Check sheet for the modelled part. Datum: model origin and axes. Units: mm. A direction names the side the tool comes from. Coordinates: 2 decimals unless noted, no trailing zeros. Loops run counter-clockwise (first coordinate to the right, second up) from the corner with the lowest first, then second, coordinate; pieces in that order, holes last. Notation, with made-up numbers: M -5,59.5 L -1,59.5 A16 ccw -1,68.5 Z; hole C 24,-22.75 d6. An arc over 180 degrees is marked long. Return JSON: item names as keys, results as strings.
from build123d import *

# Parameters (mm, degrees)
SKETCH_R      = 1.5
PAD_DEPTH     = 2.5
SKETCH001_R   = 4.25
PAD001_DEPTH  = 2.8
SKETCH002_R   = 15
PAD002_DEPTH  = 14.9
SKETCH003_R   = 2.5
PAD003_DEPTH  = 15
CHAMFER_SIZE2 = 6
CHAMFER_SIZE  = 4
SKETCH004_R   = 5
POCKET_DEPTH  = 1
SKETCH005_R   = 4
PAD004_DEPTH  = 1
SKETCH006_R   = 2
PAD005_DEPTH  = 0.95


with BuildPart() as part:
    # Sketch → Pad (new body)
    with BuildSketch(Plane.XY):
        with BuildLine():
            ThreePointArc((2.946794, 7.4375), (0, 11), (-2.946794, 7.4375))
            ThreePointArc((-3.519561, 5.765095), (-2.886811, 6.482674), (-2.946794, 7.4375))
            ThreePointArc((-3.519561, 5.765095), (-4.776172, 4.776172), (-5.765095, 3.519561))
            ThreePointArc((-7.4375, 2.946794), (-6.482674, 2.886811), (-5.765095, 3.519561))
            ThreePointArc((-7.4375, 2.946794), (-11, 0), (-7.4375, -2.946794))
            ThreePointArc((-5.765095, -3.519561), (-6.482674, -2.886811), (-7.4375, -2.946794))
            ThreePointArc((-5.765095, -3.519561), (-4.776172, -4.776172), (-3.519561, -5.765095))
            ThreePointArc((-2.946794, -7.4375), (-2.886811, -6.482674), (-3.519561, -5.765095))
            ThreePointArc((-2.946794, -7.4375), (0, -11), (2.946794, -7.4375))
            ThreePointArc((3.519561, -5.765095), (2.886811, -6.482674), (2.946794, -7.4375))
            ThreePointArc((3.519561, -5.765095), (4.776172, -4.776172), (5.765095, -3.519561))
            ThreePointArc((7.4375, -2.946794), (6.482674, -2.886811), (5.765095, -3.519561))
            ThreePointArc((7.4375, -2.946794), (11, 0), (7.4375, 2.946794))
            ThreePointArc((5.765095, 3.519561), (6.482674, 2.886811), (7.4375, 2.946794))
            ThreePointArc((5.765095, 3.519561), (4.776172, 4.776172), (3.519561, 5.765095))
            ThreePointArc((2.946794, 7.4375), (2.886811, 6.482674), (3.519561, 5.765095))
        make_face()
        with Locations((0, 8)):
            Circle(SKETCH_R, mode=Mode.SUBTRACT)
        with Locations((8, 0)):
            Circle(SKETCH_R, mode=Mode.SUBTRACT)
        with Locations((0, -8)):
            Circle(SKETCH_R, mode=Mode.SUBTRACT)
        with Locations((-8, 0)):
            Circle(SKETCH_R, mode=Mode.SUBTRACT)
    extrude(amount=PAD_DEPTH)

    # Sketch001 (on Face22 of Pad) → Pad001 (join)
    with BuildSketch(Plane.XY.offset(2.5)):
        Circle(SKETCH001_R)
    extrude(amount=PAD001_DEPTH)

    # Sketch002 (on Face24 of Pad001) → Pad002 (join)
    with BuildSketch(Plane.XY.offset(5.3)):
        Circle(SKETCH002_R)
    extrude(amount=PAD002_DEPTH)

    # Sketch003 (on Face3 of Pad002) → Pad003 (join)
    with BuildSketch(Plane.XY.offset(20.2)):
        Circle(SKETCH003_R)
    extrude(amount=PAD003_DEPTH)

    # Chamfer
    chamfer_edges = [part.edges().sort_by_distance(p)[0] for p in [
        (-15, 0, 20.2),
    ]]
    chamfer_side = part.faces().sort_by_distance((-15, 0, 12.75))[0]
    chamfer(chamfer_edges, length=CHAMFER_SIZE, length2=CHAMFER_SIZE2, reference=chamfer_side)

    # Sketch004 (on Face29 of Chamfer) → Pocket (cut)
    with BuildSketch(Plane(origin=(0, 0, 0), x_dir=(1, 0, 0), z_dir=(0, 0, -1))):
        Circle(SKETCH004_R)
    extrude(amount=-POCKET_DEPTH, mode=Mode.SUBTRACT)

    # Sketch005 (on Face31 of Pocket) → Pad004 (join)
    with BuildSketch(Plane(origin=(0, 0, 1), x_dir=(1, 0, 0), z_dir=(0, 0, -1))):
        Circle(SKETCH005_R)
    extrude(amount=PAD004_DEPTH)

    # Sketch006 (on Face33 of Pad004) → Pad005 (join)
    with BuildSketch(Plane(origin=(0, 0, 0), x_dir=(1, 0, 0), z_dir=(0, 0, -1))):
        Circle(SKETCH006_R)
    extrude(amount=PAD005_DEPTH)


solid = part.part
1) Go/stop test with flat-tipped pins: pin 1 Ø3 at (x, y) = (1, 2) entering from -Z; pin 2 Ø2.5 at (x, y) = (8, 0) entering from +Z; pin 3 Ø8 at (y, z) = (8, 12) entering from +X; pin 4 Ø2 at (x, z) = (7, 23) entering from +Y. Record where each tip stops, or that it passes through.
Answers:
{"pin 1": "z = -0.95", "pin 2": "z = 20.2", "pin 3": "x = 14.46", "pin 4": "through"}
2) Draft check along X on faces 1 (the face through (-9.5, 0.07, 1.23)), 2 (the face through (-6.47, -2.89, 1.23)), 3 (the face through (0, -11, 1)), 4 (the face through (-4.76, 4.79, 1.23)). Enter one of: +X half, -X half, draft (parallel to the pull), parting line (faces both ways), or undercut.
Answers:
{"face 1": "undercut", "face 2": "undercut", "face 3": "parting line", "face 4": "-X half"}
3) Section check A-A on x = 0. Count the separate pieces of the cut face and the enclosed holes in it, then the cut area to 3 significant figures.
Answers:
{"separate pieces": "3", "enclosed holes": "0", "area": "564 mm²"}
4) Scan lines: line 1 along Z through (x, y) = (2.75, 4); line 2 along Z through (x, y) = (-5, -5); line 3 along Y through (x, z) = (1, 4). Record each from-to range of solid material in increasing order. Write a range as [from, to].
Answers:
{"line 1": "[1, 2.5], [5.3, 20.2]", "line 2": "[5.3, 20.2]", "line 3": "[-4.13, 4.13]"}
5) Section check B-B on z = 31. Record the cut outline in (x, y).
Answers:
{"outline": "C 0,0 d5"}
6) Set-up check for faces 5 (the face through (2, -2, 20.2)), 6 (the face through (-2, 5, 0)), 7 (the face through (-2.88, -6.5, 1.23)): record each of +Z, -Z, +X, -X, +Y, -Y from which the full face is reachable in a straight line by a thin tool's end or side.
Answers:
{"face 5": "+Z", "face 6": "-Z", "face 7": "-Z, -X"}
